from build123d import *

# Parameters (mm, degrees)
SKETCH_1_R          = 12.4
SKETCH_1_R_2        = 1.6
EXTRUDE_1_DEPTH     = 19.5
EXTRUDE_START       = -10
SKETCH_4_R          = 12.4
EXTRUDE_3_DEPTH     = 10
SKETCH_5_W          = 50
SKETCH_5_H          = 36.5
EXTRUDE_4_DEPTH     = 8
SKETCH_6_W          = 152.81
SKETCH_6_H          = 50
SKETCH_6_R          = 2.6
SKETCH_6_R_2        = 1.6
EXTRUDE_5_DEPTH     = 10
SKETCH_7_R          = 4.6
CUT_EXTRUDE_1_DEPTH = 3
CHAMFER_2_SIZE      = 5
EXTRUDE_6_DEPTH     = 3
EXTRUDE_7_DEPTH     = 3
CHAMFER_3_SIZE      = 5
CHAMFER_4_SIZE      = 5
SKETCH_13_R         = 11.5
CUT_EXTRUDE_3_DEPTH = 3
CHAMFER_6_SIZE      = 1
SKETCH_18_R         = 3
CUT_EXTRUDE_6_DEPTH = 3.3


with BuildPart() as part:
    # Sketch 1 → Extrude 1 (new body)
    with BuildSketch(Plane(origin=(0, 0, 0), x_dir=(1, 0, 0), z_dir=(0, 1, 0))):
        with Locations(Location((0, 0, 0), (0, 0, 270))):
            Circle(SKETCH_1_R)
        with Locations(Location((9, 0, 0), (0, 0, 270))):
            Circle(SKETCH_1_R_2, mode=Mode.SUBTRACT)
        with Locations(Location((-4.5, -7.794228634, 0), (0, 0, 270))):
            Circle(SKETCH_1_R_2, mode=Mode.SUBTRACT)
        with Locations(Location((-4.5, 7.794228634, 0), (0, 0, 270))):
            Circle(SKETCH_1_R_2, mode=Mode.SUBTRACT)
    extrude(amount=EXTRUDE_1_DEPTH)

    # Sketch 4 → Extrude 3 (add)
    with BuildSketch(Plane(origin=(0, 19.5, 0), x_dir=(1, 0, 0), z_dir=(0, 1, 0)).offset(EXTRUDE_START)):
        with BuildLine():
            Line((0, 25), (33, 25))
            Line((33, 25), (33, -25))
            Line((33, -25), (0, -25))
            ThreePointArc((0, -25), (-25, 0), (0, 25))
        make_face()
        with Locations(Location((0, 0, 0), (0, 0, 270))):
            Circle(SKETCH_4_R, mode=Mode.SUBTRACT)
    extrude(amount=EXTRUDE_3_DEPTH)

    # Sketch 5 → Extrude 4 (add)
    with BuildSketch(Plane(origin=(33, 0, 0), x_dir=(0, 0, -1), z_dir=(1, 0, 0))):
        with Locations((0, 1.25)):
            Rectangle(SKETCH_5_W, SKETCH_5_H)
    extrude(amount=EXTRUDE_4_DEPTH)

    # Sketch 6 → Extrude 5 (add)
    with BuildSketch(Plane.XZ.offset(17)):
        with Locations((109.405, 0)):
            Rectangle(SKETCH_6_W, SKETCH_6_H)
        with Locations(Location((62.15, 0, 0), (0, 0, 270))):
            Circle(SKETCH_6_R, mode=Mode.SUBTRACT)
        with Locations(Location((156.66, 0, 0), (0, 0, 270))):
            Circle(SKETCH_6_R, mode=Mode.SUBTRACT)
        with Locations(Location((46.65, 15.5, 0), (0, 0, 270))):
            Circle(SKETCH_6_R_2, mode=Mode.SUBTRACT)
        with Locations(Location((77.65, 15.5, 0), (0, 0, 270))):
            Circle(SKETCH_6_R_2, mode=Mode.SUBTRACT)
        with Locations(Location((77.65, -15.5, 0), (0, 0, 270))):
            Circle(SKETCH_6_R_2, mode=Mode.SUBTRACT)
        with Locations(Location((46.65, -15.5, 0), (0, 0, 270))):
            Circle(SKETCH_6_R_2, mode=Mode.SUBTRACT)
        with Locations(Location((141.16, 15.5, 0), (0, 0, 270))):
            Circle(SKETCH_6_R_2, mode=Mode.SUBTRACT)
        with Locations(Location((172.16, 15.5, 0), (0, 0, 270))):
            Circle(SKETCH_6_R_2, mode=Mode.SUBTRACT)
        with Locations(Location((172.16, -15.5, 0), (0, 0, 270))):
            Circle(SKETCH_6_R_2, mode=Mode.SUBTRACT)
        with Locations(Location((141.16, -15.5, 0), (0, 0, 270))):
            Circle(SKETCH_6_R_2, mode=Mode.SUBTRACT)
    extrude(amount=EXTRUDE_5_DEPTH)

    # Sketch 7 → Cut-Extrude 1 (cut)
    with BuildSketch(Plane(origin=(0, -17, 0), x_dir=(1, 0, 0), z_dir=(0, 1, 0))):
        with Locations(Location((156.66, 0, 0), (0, 0, 270))):
            Circle(SKETCH_7_R)
    extrude(amount=-CUT_EXTRUDE_1_DEPTH, mode=Mode.SUBTRACT)

    # Chamfer 2
    chamfer_2_edges = [part.edges().sort_by_distance(p)[0] for p in [
        (-25, 19.5, 0),
        (20.5, 19.5, 25),
        (20.5, 19.5, -25),
    ]]
    chamfer(chamfer_2_edges, length=CHAMFER_2_SIZE)

    # Sketch 9 → Extrude 6 (add)
    with BuildSketch(Plane.XY.offset(25)):
        Polygon((41, 14.5), (72.5, -17), (41, -17), align=None)
    extrude(amount=-EXTRUDE_6_DEPTH)

    # Sketch 10 → Extrude 7 (add)
    with BuildSketch(Plane(origin=(0, 0, -25), x_dir=(-1, 0, 0), z_dir=(0, 0, -1))):
        Polygon((-41, -17), (-41, 14.5), (-72.5, -17), align=None)
    extrude(amount=-EXTRUDE_7_DEPTH)

    # Chamfer 3
    chamfer_3_edges = [part.edges().sort_by_distance(p)[0] for p in [
        (33, -8.75, 25),
        (33, -8.75, -25),
    ]]
    chamfer(chamfer_3_edges, length=CHAMFER_3_SIZE)

    # Chamfer 4
    chamfer_4_edges = [part.edges().sort_by_distance(p)[0] for p in [
        (185.81, -22, -25),
        (185.81, -22, 25),
    ]]
    chamfer(chamfer_4_edges, length=CHAMFER_4_SIZE)

    # Sketch 13 → Cut-Extrude 3 (cut)
    with BuildSketch(Plane(origin=(0, -17, 0), x_dir=(1, 0, 0), z_dir=(0, 1, 0))):
        with Locations(Location((62.15, 0, 0), (0, 0, 270))):
            Circle(SKETCH_13_R)
    extrude(amount=-CUT_EXTRUDE_3_DEPTH, mode=Mode.SUBTRACT)

    # Chamfer 6
    chamfer_6_edges = [part.edges().sort_by_distance(p)[0] for p in [
        (0, 0, -12.4),
    ]]
    chamfer(chamfer_6_edges, length=CHAMFER_6_SIZE)

    # Sketch 18 → Cut-Extrude 6 (cut)
    with BuildSketch(Plane(origin=(0, 19.5, 0), x_dir=(1, 0, 0), z_dir=(0, 1, 0))):
        with Locations(Location((-4.5, 7.794228634, 0), (0, 0, 270))):
            Circle(SKETCH_18_R)
        with Locations(Location((-4.5, -7.794228634, 0), (0, 0, 270))):
            Circle(SKETCH_18_R)
        with Locations(Location((9, 0, 0), (0, 0, 270))):
            Circle(SKETCH_18_R)
    extrude(amount=-CUT_EXTRUDE_6_DEPTH, mode=Mode.SUBTRACT)


solid = part.part
Can you work these out from the model? Positions are in its coordinate system, mm. A direction names the side the tool comes from. Give positions to 0.01 mm unless a question says otherwise; leave off trailing zeros. Order: outer loops, then holes, each group sorted by start corner. A loop starts at its lowest first (then second) coordinate and runs counter-clockwise, first axis right, second up. Notation, with made-up numbers: M -33.5,65 L -22.5,65 A14 ccw -22.5,82 Z; hole C -33,32.5 d6. An arc over 180 degrees is marked long. Use one line per item in the form item = value.
Item 1: If we section it at C-C, the plane y = -11: Write out the boundary of the cut face in (x, z).
Values follow:
outline = M 33,-20 L 38,-25 L 66.5,-25 L 66.5,-22 L 41,-22 L 41,22 L 66.5,22 L 66.5,25 L 38,25 L 33,20 Z
Item 2: Will these pins go through, and if not, where does the flat tip stop? pin 1 Ø5 at (x, z) = (-4.5, 7.79) entering from -Y; pin 2 Ø1.5 at (x, z) = (126, 17.5) entering from +Y; pin 3 Ø11 at (y, z) = (-14.5, -7) entering from -X; pin 4 Ø3 at (x, z) = (172.16, 15.5) entering from -Y.
Values follow:
pin_1 = 0
pin_2 = -17
pin_3 = 33
pin_4 = through
Item 3: Thinking about a two-plate mould opening in Z: for faces 5 (the flat face through (183.34, -21.93, -22.47)), 6 (the flat face through (-6, 16.2, 9)), 7 (the flat face through (183.275, -21.93, 22.535)), which applies, pulls with the +Z half, pulls with the -Z half, needs draft (parallel to the pull), parting line crosses it, or undercut?
Values follow:
face_5 = pulls with the -Z half
face_6 = undercut
face_7 = pulls with the +Z half
Item 4: If I drill on line 1 along X through (y, z) = (-21.25, 15.5); line 2 along X through (y, z) = (-19, 15); line 3 along Z through (x, y) = (156.66, -25.5), over which ranges is the centre line in solid material (lowest first)? Write a range as [from, to].
Values follow:
line_1 = [33, 45.05], [48.25, 76.05], [79.25, 139.56], [142.76, 170.56], [173.76, 185.81]
line_2 = [33, 45.13], [48.17, 76.13], [79.17, 139.64], [142.68, 170.64], [173.68, 185.81]
line_3 = [-25, -2.6], [2.6, 25]
Item 5: For faces 1 (the flat face through (35, -8, -22)), 2 (the flat face through (33, -8, 0)), 3 (the flat face through (50, -8, 22)), 4 (the cylindrical face through (161.22, -18.48, -0.6)), which set-ups out of +Z, -Z, +X, -X, +Y, -Y let a thin tool reach every point of the face, with its end or its side?
Values follow:
face_1 = -Z, -X, -Y
face_2 = +Z, -Z, -Y
face_3 = +X, +Y
face_4 = +Y
Item 6: If we section it at D-D, the plane x = 168: Write out the boundary of the cut face in (y, z), and give its area (3 significant figures).
Values follow:
outline = M -27,-25 L -17,-25 L -17,25 L -27,25 Z
area = 500 mm^2
Item 7: If we section it at A-A, the plane x = 62.15: Write out the boundary of the cut face in (y, z), and give its area (3 significant figures).
Values follow:
outline = M -27,-25 L -6.65,-25 L -6.65,-22 L -17,-22 L -17,-11.5 L -20,-11.5 L -20,-2.6 L -27,-2.6 Z; M -27,2.6 L -20,2.6 L -20,11.5 L -17,11.5 L -17,22 L -6.65,22 L -6.65,25 L -27,25 Z
area = 457 mm^2
Item 8: If we section it at B-B, the plane y = -23: Count the separate pieces of the cut face and the enclosed holes in it, and give its area (3 significant figures).
Values follow:
separate_pieces = 1
enclosed_holes = 10
area = 7,480 mm^2
